For this review, take the finished solid that the model builds, in its own axes (mm). Face numbers are marked on the shaded views. Coordinates: 2 decimals unless noted, no trailing zeros. Write each loop counter-clockwise with the first axis right and the second up, starting at its lowest first coordinate (ties: lowest second). Pieces come first, ordered by that corner, then holes.
```python
from build123d import *

# Parameters (mm, degrees)
BOSS_EXTRUDE1_DEPTH = 9.525
FILLET1_R           = 2.54
SKETCH2_R           = 12.3825
CUT_EXTRUDE1_DEPTH  = 10.525
FILLET2_R           = 1.27


with BuildPart() as part:
    # Sketch1 → Boss-Extrude1 (new body)
    with BuildSketch(Plane.XY):
        Polygon((-7.339781299, 15.8115), (7.339781299, 15.8115), (15.8115, 6.35), (15.8115, -6.35), (7.339781299, -15.8115), (-7.339781299, -15.8115), (-15.8115, -6.35), (-15.8115, 6.35), align=None)
    extrude(amount=BOSS_EXTRUDE1_DEPTH)

    # Fillet1
    fillet1_edges = [part.edges().sort_by_distance(p)[0] for p in [
        (15.8115, 0, 0),
        (11.575640649, -11.08075, 0),
        (0, -15.8115, 0),
        (-11.575640649, -11.08075, 0),
        (-15.8115, 0, 0),
        (-11.575640649, 11.08075, 0),
        (0, 15.8115, 0),
        (11.575640649, 11.08075, 0),
    ]]
    fillet(fillet1_edges, radius=FILLET1_R)

    # Sketch2 → Cut-Extrude1 (cut, through all)
    with BuildSketch(Plane(origin=(0, 0, 0), x_dir=(-1, 0, 0), z_dir=(0, 0, -1))):
        Circle(SKETCH2_R)
    extrude(amount=-CUT_EXTRUDE1_DEPTH, mode=Mode.SUBTRACT)

    # Fillet2
    fillet2_edges = [part.edges().sort_by_distance(p)[0] for p in [
        (11.575640649, -11.08075, 9.525),
        (15.8115, 0, 9.525),
        (11.575640649, 11.08075, 9.525),
        (0, 15.8115, 9.525),
        (-11.575640649, 11.08075, 9.525),
        (-15.8115, 0, 9.525),
        (-11.575640649, -11.08075, 9.525),
        (0, -15.8115, 9.525),
    ]]
    fillet(fillet2_edges, radius=FILLET2_R)


solid = part.part
```
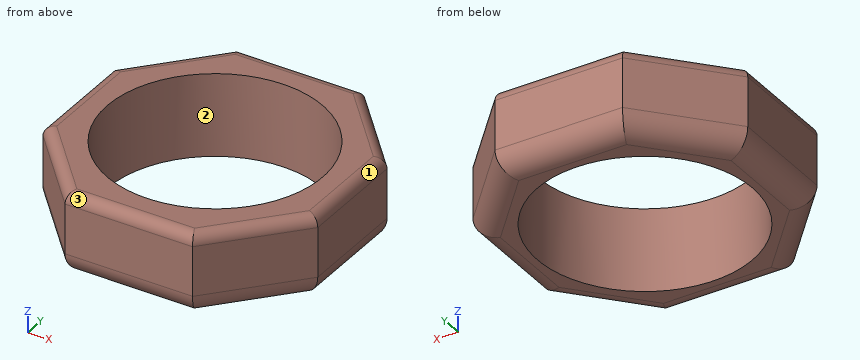
Q1. Add section D-D (z = 2). State the section outline as (x, y) points (1 decimal), then the cut area to 3 significant figures.
Ans:
outline: (-15.8, -6.3) - (-7.3, -15.8) - (7.3, -15.8) - (15.8, -6.3) - (15.8, 6.3) - (7.3, 15.8) - (-7.3, 15.8) - (-15.8, 6.3) - close; hole circle Ø24.8 at (0, 0)
area: 352 mm2
Q2. Draft analysis for pull direction X (two halves, no side actions). For the marked faces 1, 2 and 3, state which applies: +X half, -X half, draft (parallel to the pull), parting line (faces both ways), or undercut.
Ans:
face 1: +X half
face 2: undercut
face 3: draft
Q3. For probe 1 along Y at (x, z) = (0, 6.25); probe 2 along X at (y, z) = (1.5, 8.5); probe 3 along Y at (x, z) = (-2, 3.5), list the stretches that pass through material, from the lowest coordinate up.
Ans:
probe 1: y = -15.81 to -12.38, 12.38 to 15.81
probe 2: x = -15.79 to -12.29, 12.29 to 15.79
probe 3: y = -15.81 to -12.22, 12.22 to 15.81
Q4. Add section A-A (x = 0). State the section outline as (y, z) points (1 decimal), then the cut area to 3 significant figures.
Ans:
outline: (-15.8, 2.5) arc R2.5 ccw to (-13.3, 0) - (-12.4, 0) - (-12.4, 9.5) - (-14.5, 9.5) arc R1.3 ccw to (-15.8, 8.3) - close; (12.4, 0) - (13.3, 0) arc R2.5 ccw to (15.8, 2.5) - (15.8, 8.3) arc R1.3 ccw to (14.5, 9.5) - (12.4, 9.5) - close
area: 61.9 mm2
Q5. Clearance check with flat-ended pins moving along their axes: pin 1 Ø1 at (y, z) = (0, 1.5) entering from -X; pin 2 Ø1 at (x, z) = (12.5, 2.5) entering from -Y. State where each tip first meets the part, or that it passes through.
Ans:
pin 1: stops at x = -15.75
pin 2: stops at y = -10.61
